Can you work these out from the model? Positions are in its coordinate system, mm. A direction names the side the tool comes from. Coordinates: 2 decimals unless noted, no trailing zeros. Order: outer loops, then holes, each group sorted by start corner. A loop starts at its lowest first (then second) coordinate and runs counter-clockwise, first axis right, second up. Notation, with made-up numbers: (2, 10.25) -> (14, 10.25) arc R17 cw to (14, 15.25) -> close; hole circle Ø8 at (58, 73). An arc over 180 degrees is marked (long way). Write item = value, one per line.
```python
from build123d import *

# Parameters (mm, degrees)
F0_W           = 120
F0_H           = 30
F0_R           = 5
F1_DEPTH       = 10
F3_D           = 8
F3_CBORE_D     = 11.25
F3_CBORE_DEPTH = 6
F5_D           = 4


with BuildPart() as f1:
    # F0 (on Top) → F1 (new body)
    with BuildSketch(Plane.XY):
        with Locations((-15, 0)):
            Rectangle(F0_W, F0_H)
        Circle(F0_R, mode=Mode.SUBTRACT)
    extrude(amount=F1_DEPTH)

    # F3 (through all)
    with Locations(Plane(origin=(0, 0, 0), x_dir=(1, 0, 0), z_dir=(0, 0, -1))):
        with Locations((-65, 8), (-65, -8)):
            CounterBoreHole(F3_D / 2, F3_CBORE_D / 2, F3_CBORE_DEPTH)

    # F5 (through all)
    with Locations(Plane.XY.offset(10)):
        with Locations((-33, 0)):
            Hole(F5_D / 2)


solid = f1.part
```
Item 1: I want a section at B-B, the plane x = 0. Please give me the cut outline in (y, z).
A:
outline = (-15, 0) -> (-5, 0) -> (-5, 10) -> (-15, 10) -> close; (5, 0) -> (15, 0) -> (15, 10) -> (5, 10) -> close
Item 2: I want a section at D-D, the plane y = 0. Please give me the cut outline in (x, z).
A:
outline = (-75, 0) -> (-35, 0) -> (-35, 10) -> (-75, 10) -> close; (-31, 0) -> (-5, 0) -> (-5, 10) -> (-31, 10) -> close; (5, 0) -> (45, 0) -> (45, 10) -> (5, 10) -> close
Item 3: I'm going to push flat-ended pins straight in: P1, Ø5.5, axis at x = -67, y = -6, coming from the -Z side; P2, Ø6.5, axis at x = -65, y = 8, coming from the +Z side. Where does each tip first touch, or does it pass through?
A:
P1 = 6
P2 = through
Item 4: If we mould it in two halves opening along Y, with no side actions, what happens to faces 3 (the flat face through (-16, -15, 5)), 4 (the flat face through (-16, 0, 0)), 5 (the cylindrical face through (-68.695, 9.532, 8.028))? For each: pulls with the +Y half, pulls with the -Y half, needs draft (parallel to the pull), parting line crosses it, or undercut.
A:
face_3 = pulls with the -Y half
face_4 = needs draft
face_5 = undercut
Item 5: If I drill on probe 1 along Y at (x, z) = (-65, 3.6) (3 decimals); probe 2 along Y at (x, z) = (-65, 8.55); probe 3 along Y at (x, z) = (0, 4), over which ranges is the centre line in solid material (lowest first)?
A:
probe_1 = -15 to -13.625, -2.375 to 2.375, 13.625 to 15
probe_2 = -15 to -12, -4 to 4, 12 to 15
probe_3 = -15 to -5, 5 to 15
Item 6: I want a section at C-C, the plane z = 3.75. Please give me the cut outline in (x, y) (3 decimals).
A:
outline = (-75, -15) -> (45, -15) -> (45, 15) -> (-75, 15) -> close; hole circle Ø11.25 at (-65, -8); hole circle Ø11.25 at (-65, 8); hole circle Ø4 at (-33, 0); hole circle Ø10 at (0, 0)
Item 7: I want a section at A-A, the plane y = -8. Please give me the cut outline in (x, z) (3 decimals), plus the area to 3 significant figures.
A:
outline = (-75, 0) -> (-70.625, 0) -> (-70.625, 6) -> (-69, 6) -> (-69, 10) -> (-75, 10) -> close; (-61, 6) -> (-59.375, 6) -> (-59.375, 0) -> (45, 0) -> (45, 10) -> (-61, 10) -> close
area = 1,100 mm2
Item 8: For faces 1 (the flat face through (-16, 15, 5)), 2 (the cylindrical face through (-59.8, -5.85, 2.96)), which set-ups out of +Z, -Z, +X, -X, +Y, -Y let a thin tool reach every point of the face, with its end or its side?
A:
face_1 = +Z, -Z, +X, -X, +Y
face_2 = -Z
